```python
from build123d import *

# Parameters (mm, degrees)
F0_W     = 125
F0_H     = 50
F1_DEPTH = 11
F3_DEPTH = 8
F5_DEPTH = 5
F7_D     = 8
F7_DEPTH = 10.6
F7_TIP   = 2.4034424761
F9_D     = 8
F9_DEPTH = 10.6
F9_TIP   = 2.4034424761


with BuildPart() as f1:
    # F0 (on Top) → F1 (new body)
    with BuildSketch(Plane.XY):
        Rectangle(F0_W, F0_H)
    extrude(amount=F1_DEPTH)

    # F2 (on face) → F3 (join)
    with BuildSketch(Plane.XY.offset(11)):
        with BuildLine():
            ThreePointArc((37.5, -20), (57.5, 0), (37.5, 20))
            Line((37.5, 20), (-37.5, 20))
            ThreePointArc((-37.5, 20), (-57.5, 0), (-37.5, -20))
            Line((-37.5, -20), (37.5, -20))
        make_face()
    extrude(amount=F3_DEPTH)

    # F4 (on face) → F5 (cut)
    with BuildSketch(Plane.XY.offset(19)):
        with BuildLine():
            ThreePointArc((37.5, -6), (43.5, 0), (37.5, 6))
            Line((37.5, 6), (-37.5, 6))
            ThreePointArc((-37.5, 6), (-43.5, 0), (-37.5, -6))
            Line((-37.5, -6), (37.5, -6))
        make_face()
    extrude(amount=-F5_DEPTH, mode=Mode.SUBTRACT)

    # F7
    with Locations(Plane.XY.offset(14)):
        with Locations((0, 0)):
            Hole(F7_D / 2, depth=F7_DEPTH)
            with Locations((0, 0, -(F7_DEPTH + F7_TIP / 2))):  # 118° drill point
                Cone(0, F7_D / 2, F7_TIP, mode=Mode.SUBTRACT)

    # F9
    with Locations(Plane.XY.offset(14)):
        with Locations((-37.5, 0), (37.5, 0)):
            Hole(F9_D / 2, depth=F9_DEPTH)
            with Locations((0, 0, -(F9_DEPTH + F9_TIP / 2))):  # 118° drill point
                Cone(0, F9_D / 2, F9_TIP, mode=Mode.SUBTRACT)


solid = f1.part
```
Input: part model. Units: mm. Frame: model coordinates. A direction names the side the tool comes from. Give positions to 0.01 mm unless a question says otherwise; leave off trailing zeros. Write each loop counter-clockwise with the first axis right and the second up, starting at its lowest first coordinate (ties: lowest second). Pieces come first, ordered by that corner, then holes. Notation, with made-up numbers: (74, -27.5) - (82, -27.5) arc R29 cw to (82, -3.5) - close; hole circle Ø11 at (-28.75, 85.25). An arc over 180 degrees is marked (long way). Write item = value, one per line. Start each with the question number.
1) Cut plane A-A (z = 12.75). Return loops of the section in (x, y), and give its area (3 significant figures).
2) Cut plane B-B (x = -16.5). Return loops of the section in (y, z).
3) Pin query (flat end, axial travel): pin 1 (10.5 mm diameter, centred on x = 0, y = 0, fed in from +Z); pin 2 (2.5 mm diameter, centred on x = -15, z = 16.5, fed in from -Y); pin 3 (1.5 mm diameter, centred on x = -18.5, z = 15.5, fed in from +Y). Return the tip coordinate at first contact, or that it passes through.
4) Material intervals for L1, parallel to X at y = 0, z = 7; L2, parallel to X at y = 0, z = 11.25; L3, parallel to Y at x = 37.5, z = 6.5, sorted ascending. Write a range as [from, to].
5) Reachability of faces 1 (the face through (57.495, -0.44, 14.944)), 2 (the face through (1, 6, 17)), 3 (the face through (-57.495, 0.44, 14.944)), 4 (the face through (1, 20, 15)) from +Z, -Z, +X, -X, +Y, -Y: full face, straight path, thin tool, end or side. Return the list, or none.
6) Draft query along X for faces 5 (the face through (-1, -25, 5)), 6 (the face through (-62.5, 0, 5)), 7 (the face through (43.5, -0.1, 16.5)), 8 (the face through (-1, -6, 17)). Return one class per face: pulls with the +X half, pulls with the -X half, needs draft (parallel to the pull), parting line crosses it, or undercut.
Answers follow:
q1.outline = (-37.5, -20) - (37.5, -20) arc R20 ccw to (37.5, 20) - (-37.5, 20) arc R20 ccw to start; hole circle Ø8 at (-37.5, 0); hole circle Ø8 at (0, 0); hole circle Ø8 at (37.5, 0)
q1.area = 4,110 mm^2
q2.outline = (-25, 0) - (25, 0) - (25, 11) - (20, 11) - (20, 19) - (6, 19) - (6, 14) - (-6, 14) - (-6, 19) - (-20, 19) - (-20, 11) - (-25, 11) - close
q3.pin_1 = 14
q3.pin_2 = -20
q3.pin_3 = 20
q4.L1 = [-62.5, -41.5], [-33.5, -4], [4, 33.5], [41.5, 62.5]
q4.L2 = [-57.5, -41.5], [-33.5, -4], [4, 33.5], [41.5, 57.5]
q4.L3 = [-25, -4], [4, 25]
q5.face_1 = +Z, +X
q5.face_2 = +Z
q5.face_3 = +Z, -X
q5.face_4 = +Z, +X, -X, +Y
q6.face_5 = needs draft
q6.face_6 = pulls with the -X half
q6.face_7 = undercut
q6.face_8 = undercut
